from build123d import *

# Parameters (mm, degrees)
CUT_EXTRUDE_1_DEPTH = 156.307191324


with BuildPart() as part:
    # По траектории1: sweep along a path in Эскиз2
    with BuildLine(Plane(origin=(0, 0, 0), x_dir=(1, 0, 0), z_dir=(0, 1, 0))) as sweep_1_path:
        Line((-19.053699061, 0), (-19.053699061, 130))
        ThreePointArc((-19.053699061, 130), (-1.553699061, 147.5), (15.946300939, 130))
        Line((15.946300939, 130), (15.946300939, 0))
    # Эскиз1 → По траектории1 (sweep)
    with BuildSketch(Plane.XY):
        with BuildLine():
            Line((-19.103699061, 0.491825411), (-19.003699061, 0.491825411))
            ThreePointArc((-19.003699061, 0.491825411), (-17.271287447, -0.225762975), (-16.553699061, -1.958174589))
            Line((-16.553699061, -1.958174589), (-16.553699061, -2.058174589))
            ThreePointArc((-16.553699061, -2.058174589), (-17.271287447, -3.790586203), (-19.003699061, -4.508174589))
            Line((-19.003699061, -4.508174589), (-19.103699061, -4.508174589))
            ThreePointArc((-19.103699061, -4.508174589), (-20.836110675, -3.790586203), (-21.553699061, -2.058174589))
            Line((-21.553699061, -2.058174589), (-21.553699061, -1.958174589))
            ThreePointArc((-21.553699061, -1.958174589), (-20.836110675, -0.225762975), (-19.103699061, 0.491825411))
        make_face()
    sweep(path=sweep_1_path.line)

    # Эскиз3 → Вырез-Вытянуть1 (cut, through all)
    with BuildSketch(Plane.ZY.offset(21.553699061)):
        Polygon((0, 0.491825411), (-5, 0.491825411), (0, -4.508174589), align=None)
    extrude(amount=-CUT_EXTRUDE_1_DEPTH, mode=Mode.SUBTRACT)


solid = part.part
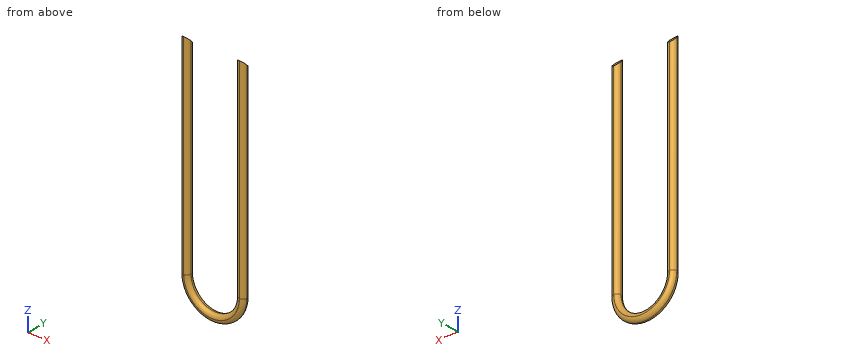
Design review of the part built by this model. Coordinates are the model's own, in mm. Round coordinates to 2 decimals unless told otherwise and drop trailing zeros. Write each loop counter-clockwise with the first axis right and the second up, starting at its lowest first coordinate (ties: lowest second). Pieces come first, ordered by that corner, then holes.
Item 1: Wall thickness on L1, parallel to X at y = -3.7, z = -135; L2, parallel to X at y = -3.8, z = -88.5; L3, parallel to Z at x = -11.5, y = -4.2: over which ranges is each line inside the solid? List them lowest first.
Item 2: Consider section A-A on z = -63.5. Give the boundary of the cut face in (x, y), and give its area (3 significant figures).
Item 3: For pin 1 Ø1 at (x, y) = (0.5, -4) entering from +Z; pin 2 Ø2 at (y, z) = (-3, -81) entering from -X; pin 3 Ø1.5 at (y, z) = (-3.5, -63) entering from +X; pin 4 Ø1 at (x, y) = (-11, -2.5) entering from +Z, all flat-tipped, find the tip position at first contact; note any pin that passes through.
Item 4: Consider section B-B on y = -0.4. Give the boundary of the cut face in (x, z), and give its area (3 significant figures).
Check values:
1. L1: x = -20.27 to -16.36, 13.26 to 17.16
1. L2: x = -20.83 to -17.28, 14.17 to 17.72
1. L3: z = -145.88 to -142.86
2. outline: (-21.55, -2.06) arc R2.45 ccw to (-19.1, -4.51) - (-19, -4.51) arc R2.45 ccw to (-16.55, -2.06) - (-16.55, -1.96) arc R2.45 ccw to (-19, 0.49) - (-19.1, 0.49) arc R2.45 ccw to (-21.55, -1.96) - close; (13.45, -2.06) arc R2.45 ccw to (15.9, -4.51) - (16, -4.51) arc R2.45 ccw to (18.45, -2.06) - (18.45, -1.96) arc R2.45 ccw to (16, 0.49) - (15.9, 0.49) arc R2.45 ccw to (13.45, -1.96) - close
2. area: 39.7 mm2
3. pin 1: stops at z = -145.33
3. pin 2: stops at x = -21.55
3. pin 3: stops at x = 18.35
3. pin 4: stops at z = -141.27
4. outline: (-20.99, -130) arc R19.44 ccw to (17.89, -130) - (17.89, -4.11) - (14.01, -4.11) - (14.01, -130) arc R15.56 cw to (-17.11, -130) - (-17.11, -4.11) - (-20.99, -4.11) - close
4. area: 1,190 mm2
